Part print with two shaded views. Sizes in mm from the minimum x, y, z corner. Give positions to 0.01 mm unless a question says otherwise; leave off trailing zeros. Order: outer loops, then holes, each group sorted by start corner. A loop starts at its lowest first (then second) coordinate and runs counter-clockwise, first axis right, second up. Notation, with made-up numbers: (-35, 22.25) -> (-11, 22.25) arc R27 ccw to (-11, 46.25) -> close; hole circle Ø7 at (27.25, 44.25). An arc over 180 degrees is marked (long way). Answer in a Markdown table with one row per item. Add a question column.
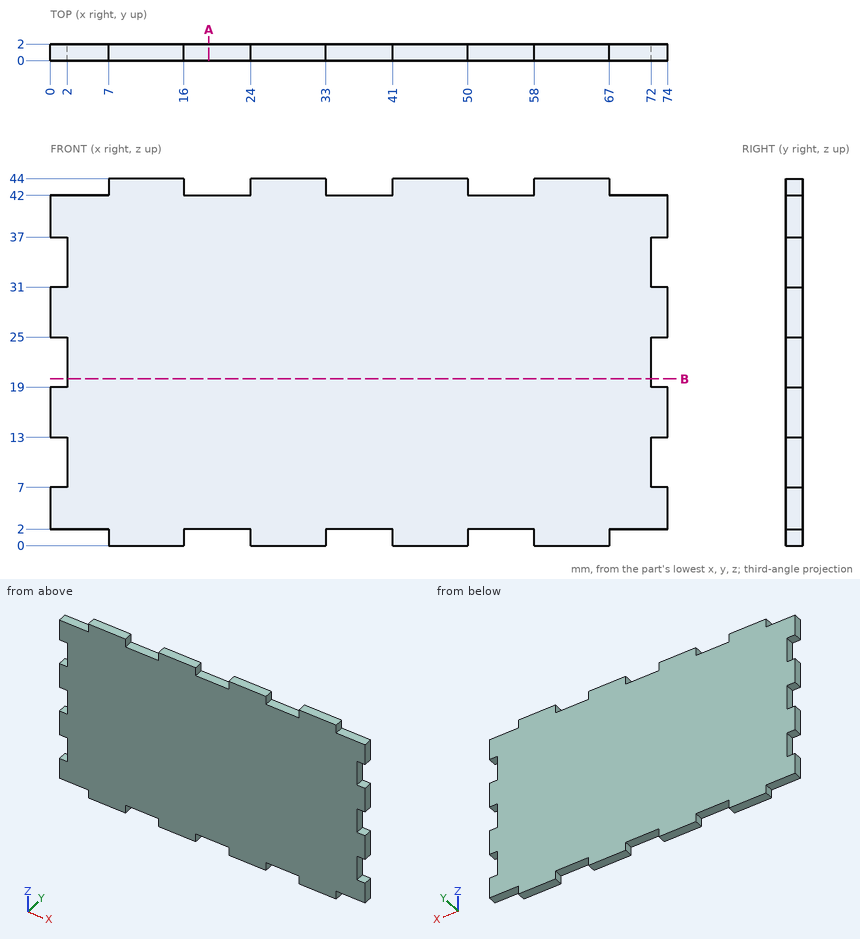
Item 1: Pin check, flat tips, straight feed: pin 1 Ø0.6 at (x, y) = (18.5, 1.5) entering from -Z; pin 2 Ø1 at (x, y) = (18.5, 1.5) entering from +Z. Stop position of each tip, or through.
Item 2: Saw through at A-A on x = 19. List the corners of the cut face in (y, z).
Item 3: Wall check: line 1 (Z direction, x = 38.5, y = 0.25); line 2 (X direction, y = 1.5, z = 12). Give the ranges that are in metal, low to high.
Item 4: Saw through at B-B on z = 20. List the corners of the cut face in (x, y).
Evaluation:
| question | item | result |
|---|---|---|
| 1 | pin 1 | stops at z = 2 |
| 1 | pin 2 | stops at z = 42 |
| 2 | outline | (0, 2) -> (2, 2) -> (2, 42) -> (0, 42) -> close |
| 3 | line 1 | z = 2 to 42 |
| 3 | line 2 | x = 2 to 72 |
| 4 | outline | (2, 0) -> (72, 0) -> (72, 2) -> (2, 2) -> close |
